Input: part model. Units: mm. Frame: model coordinates. Face numbers are marked on the shaded views. A direction names the side the tool comes from. Give positions to 0.01 mm unless a question says otherwise; leave off trailing zeros. Loops run counter-clockwise (first coordinate to the right, second up) from the corner with the lowest first, then second, coordinate; pieces in that order, holes last. Notation, with made-up numbers: (19.5, 17) - (71.5, 17) arc R26 ccw to (71.5, 52) - close; hole circle Ø1 at (52.25, -25.5). An arc over 180 degrees is marked (long way). One line per item, written item: value.
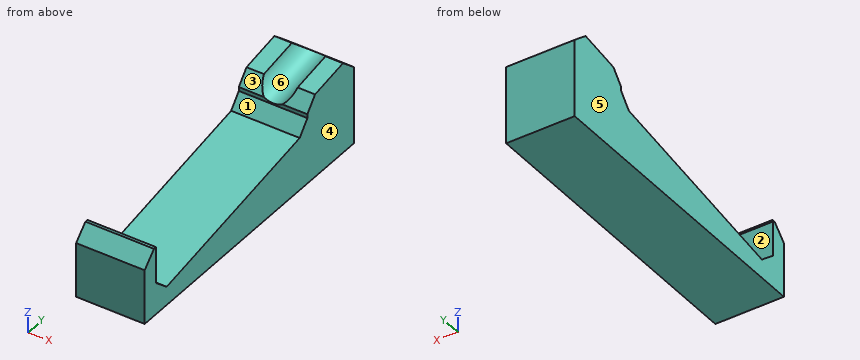
from build123d import *

# Parameters (mm, degrees)
F1_DEPTH     = 12.7
F3_R         = 6.35
F4_DEPTH     = 104.14
F5_T1_DEPTH  = 25.4
F5_T3_DEPTH  = 51.5282991577
F5_T5_DEPTH  = 37.3912990947
F5_T7_DEPTH  = 28.55897566
F5_T9_DEPTH  = 28.55897566
F5_T11_DEPTH = 37.3912990947


# Not quite as in the source:
# - a fillet or chamfer that OpenCascade refuses, or shapes differently, is made with other operations: its cross-section is extruded or revolved along the edge and cut away or added


with BuildPart() as f1:
    # F0 (on Right) → F1 (new body, symmetric)
    with BuildSketch(Plane.YZ):
        Polygon((-114.3, 25.4), (-114.3, 0), (0, 0), (0, 34.925), (-25.4, 30.44629469), (-25.4, 20.4565655141), (-108.2500742316, 5.8478620733), (-108.2500742316, 24.8292279061), (-108.1259697676, 24.8511108716), (-108.1259697676, 25.4), align=None)
    extrude(amount=F1_DEPTH, both=True)

    # F3 (on face) → F4 (cut)
    with BuildSketch(Plane(origin=(0, 5.9725267528, 1.0531176095), x_dir=(1, 0, 0), z_dir=(0, -0.984807753, -0.1736481777))):
        with Locations((0, 35.56)):
            Circle(F3_R)
    extrude(amount=F4_DEPTH, mode=Mode.SUBTRACT)

    # F5: chamfer of 5.08 on 7 edges, made by hand

    # F5_s2 → F5_t1 (join)
    with BuildSketch(Plane.YZ.offset(-12.7)):
        Polygon((-25.4, 24.7191916404), (-29.5978672575, 19.7163682551), (-25.4, 20.4565655141), align=None)
        Polygon((-102.2879414891, 6.8991469384), (-108.2500742316, 11.9019703237), (-108.2500742316, 5.8478620733), align=None)
    extrude(amount=F5_T1_DEPTH)

    # F5_s4 → F5_t3 (cut)
    with BuildSketch(Plane.YZ.offset(-25.7641495789)):
        Polygon((-114.3, 20.32), (-109.22, 25.4), (-114.3, 25.4), align=None)
    extrude(amount=F5_T3_DEPTH, mode=Mode.SUBTRACT)

    # F5_s6 → F5_t5 (cut)
    with BuildSketch(Plane.YZ.offset(-28.1667031257)):
        Polygon((0, 28.8708917496), (-5.9621327425, 33.8737151349), (0, 34.925), align=None)
    extrude(amount=F5_T5_DEPTH, mode=Mode.SUBTRACT)

    # F5_s8 → F5_t7 (cut)
    with BuildSketch(Plane.YZ.offset(-4.8084342517)):
        Polygon((-25.4, 26.1836685636), (-21.2021327425, 31.1864919489), (-25.4, 30.44629469), align=None)
    extrude(amount=F5_T7_DEPTH, mode=Mode.SUBTRACT)

    # F5_s10 → F5_t9 (cut)
    with BuildSketch(Plane.YZ.offset(-23.7505414084)):
        Polygon((-21.2021327425, 31.1864919489), (-25.4, 26.1836685636), (-25.4, 30.44629469), align=None)
    extrude(amount=F5_T9_DEPTH, mode=Mode.SUBTRACT)

    # F5_s12 → F5_t11 (cut)
    with BuildSketch(Plane.YZ.offset(-9.224595969)):
        Polygon((0, 28.8708917496), (-5.9621327425, 33.8737151349), (0, 34.925), align=None)
    extrude(amount=F5_T11_DEPTH, mode=Mode.SUBTRACT)


solid = f1.part
Item 1: Draft query along X for the marked faces 4, 5 and 6. Return one class per face: pulls with the +X half, pulls with the -X half, needs draft (parallel to the pull), parting line crosses it, or undercut.
Verdict:
face 4: pulls with the +X half
face 5: pulls with the -X half
face 6: undercut
Item 2: Section D-D, the plane x = -1.25. Output: boundary loops of the cut face in (y, z), and give its area (3 significant figures).
Verdict:
outline: (-114.3, 0) - (0, 0) - (0, 28.87) - (-0.9, 29.63) - (-25.4, 25.31) - (-25.4, 24.72) - (-29.6, 19.72) - (-102.29, 6.9) - (-108.25, 11.9) - (-108.25, 24.83) - (-108.13, 24.85) - (-108.13, 25.4) - (-109.22, 25.4) - (-114.3, 20.32) - close
area: 1,960 mm^2
Item 3: Material intervals for L1, parallel to Y at x = 6.5, z = 20; L2, parallel to Z at x = -0.25, y = -108.5; L3, parallel to Y at x = 2.5, z = 23.5, sorted ascending.
Verdict:
L1: y = -114.3 to -108.25, -29.36 to 0
L2: z = 0 to 25.4
L3: y = -111.12 to -108.25, -26.42 to 0
Item 4: Access query for the marked faces 1, 2 and 3. Directions: +Z, -Z, +X, -X, +Y, -Y. A direction counts if a zero-diameter tool reaches every point of the face in a straight line with its end or side. Return the directions, or none.
Verdict:
face 1: +Z, +X, -X
face 2: +X, -X
face 3: +Z, +X, -X, -Y
Item 5: Section C-C, the plane y = -59.5. Output: boundary loops of the cut face in (x, z).
Verdict:
outline: (-12.7, 0) - (12.7, 0) - (12.7, 14.44) - (-12.7, 14.44) - close
Item 6: Section B-B, the plane z = 16. Output: boundary loops of the cut face in (x, y).
Verdict:
outline: (-12.7, -114.3) - (12.7, -114.3) - (12.7, -108.25) - (-12.7, -108.25) - close; (-12.7, -50.67) - (12.7, -50.67) - (12.7, 0) - (-12.7, 0) - close
Item 7: Pin query (flat end, axial travel): P1, Ø4, axis at x = -3.5, y = -23, coming from the +Z side; P2, Ø0.5, axis at x = -2.5, y = -108.5, coming from the +Z side; P3, Ø5, axis at x = 0, y = -43, coming from the +Z side. Return the tip coordinate at first contact, or that it passes through.
Verdict:
P1: stops at z = 28.85
P2: stops at z = 25.4
P3: stops at z = 17.79
Item 8: Section A-A, the plane x = -9. Output: boundary loops of the cut face in (y, z), and give its area (3 significant figures).
Verdict:
outline: (-114.3, 0) - (0, 0) - (0, 28.87) - (-5.96, 33.87) - (-21.2, 31.19) - (-25.4, 26.18) - (-25.4, 24.72) - (-29.6, 19.72) - (-102.29, 6.9) - (-108.25, 11.9) - (-108.25, 24.83) - (-108.13, 24.85) - (-108.13, 25.4) - (-109.22, 25.4) - (-114.3, 20.32) - close
area: 2,060 mm^2
